Check sheet for the modelled part. Datum: model origin and axes. Units: mm. A direction names the side the tool comes from. Coordinates: 2 decimals unless noted, no trailing zeros. Loops run counter-clockwise (first coordinate to the right, second up) from the corner with the lowest first, then second, coordinate; pieces in that order, holes last. Notation, with made-up numbers: M 68.5,72 L 75.5,72 A9 ccw 75.5,79 Z; hole C 80,80 d10. An arc over 180 degrees is marked long. Return JSON: item names as keys, results as strings.
from build123d import *

# Parameters (mm, degrees)
SKETCH1_W           = 285
SKETCH1_H           = 36
SKETCH1_R           = 1.5
SKETCH1_W_2         = 42
SKETCH1_H_2         = 20
BOSS_EXTRUDE2_DEPTH = 5
FILLET1_R           = 6
FILLET2_R           = 1


with BuildPart() as part:
    # Sketch1 → Boss-Extrude2 (new body)
    with BuildSketch(Plane(origin=(0, 0, 0), x_dir=(1, 0, 0), z_dir=(0, 1, 0))):
        Rectangle(SKETCH1_W, SKETCH1_H)
        with Locations(Location((-22.5, -12, 0), (0, 0, 270))):
            Circle(SKETCH1_R, mode=Mode.SUBTRACT)
        with Locations(Location((-22.5, 12, 0), (0, 0, 90))):
            Circle(SKETCH1_R, mode=Mode.SUBTRACT)
        with Locations(Location((-136.5, -12, 0), (0, 0, 270))):
            Circle(SKETCH1_R, mode=Mode.SUBTRACT)
        with Locations(Location((-136.5, 12, 0), (0, 0, 90))):
            Circle(SKETCH1_R, mode=Mode.SUBTRACT)
        with Locations(Location((22.5, -12, 0), (0, 0, 90))):
            Circle(SKETCH1_R, mode=Mode.SUBTRACT)
        with Locations(Location((22.5, 12, 0), (0, 0, 270))):
            Circle(SKETCH1_R, mode=Mode.SUBTRACT)
        with Locations(Location((136.5, -12, 0), (0, 0, 90))):
            Circle(SKETCH1_R, mode=Mode.SUBTRACT)
        with Locations(Location((136.5, 12, 0), (0, 0, 270))):
            Circle(SKETCH1_R, mode=Mode.SUBTRACT)
        with Locations(Location((-60, 12, 0), (0, 0, 270))):
            Circle(SKETCH1_R, mode=Mode.SUBTRACT)
        with Locations(Location((-60, -12, 0), (0, 0, 90))):
            Circle(SKETCH1_R, mode=Mode.SUBTRACT)
        with Locations(Location((60, -12, 0), (0, 0, 270))):
            Circle(SKETCH1_R, mode=Mode.SUBTRACT)
        with Locations(Location((60, 12, 0), (0, 0, 90))):
            Circle(SKETCH1_R, mode=Mode.SUBTRACT)
        with Locations((-109, 0)):
            Rectangle(SKETCH1_W_2, SKETCH1_H_2, mode=Mode.SUBTRACT)
        with Locations((109, 0)):
            Rectangle(SKETCH1_W_2, SKETCH1_H_2, mode=Mode.SUBTRACT)
    extrude(amount=BOSS_EXTRUDE2_DEPTH)

    # Fillet1
    fillet1_edges = [part.edges().sort_by_distance(p)[0] for p in [
        (142.5, 2.5, 18),
        (-142.5, 2.5, 18),
        (-142.5, 2.5, -18),
        (142.5, 2.5, -18),
    ]]
    fillet(fillet1_edges, radius=FILLET1_R)

    # Fillet2
    fillet2_edges = [part.edges().sort_by_distance(p)[0] for p in [
        (-88, 2.5, 10),
        (-88, 2.5, -10),
        (-130, 2.5, -10),
        (-130, 2.5, 10),
        (88, 2.5, -10),
        (88, 2.5, 10),
        (130, 2.5, 10),
        (130, 2.5, -10),
    ]]
    fillet(fillet2_edges, radius=FILLET2_R)


solid = part.part
1) Set-up check for faces 5 (the face through (142.5, 2, 0)), 6 (the face through (-88, 2, 0)): record each of +Z, -Z, +X, -X, +Y, -Y from which the full face is reachable in a straight line by a thin tool's end or side.
Answers:
{"face 5": "+Z, -Z, +X, +Y, -Y", "face 6": "+Y, -Y"}
2) Draft check along Z on faces 1 (the face through (-2, 0, 0)), 2 (the face through (140.696, 2.535, 16.289)), 3 (the face through (-109, 2, -10)), 4 (the face through (109, 2, 10)). Enter one of: +Z half, -Z half, draft (parallel to the pull), parting line (faces both ways), or undercut.
Answers:
{"face 1": "draft", "face 2": "+Z half", "face 3": "undercut", "face 4": "undercut"}
3) Section check A-A on x = -96. Record the cut outline in (y, z).
Answers:
{"outline": "M 0,-18 L 5,-18 L 5,-10 L 0,-10 Z; M 0,10 L 5,10 L 5,18 L 0,18 Z"}
4) Scan lines: line 1 along X through (y, z) = (0.45, 7); line 2 along Z through (x, y) = (136.5, 3.55); line 3 along Z through (x, y) = (-116, 0.85). Record each from-to range of solid material in increasing order. Write a range as [from, to].
Answers:
{"line 1": "[-142.5, -130], [-88, 88], [130, 142.5]", "line 2": "[-18, -13.5], [-10.5, 10.5], [13.5, 18]", "line 3": "[-18, -10], [10, 18]"}
5) Go/stop test with flat-tipped pins: pin 1 Ø1.8 at (x, z) = (-136.5, -12) entering from -Y; pin 2 Ø5 at (x, z) = (136.5, 12) entering from -Y. Record where each tip stops, or that it passes through.
Answers:
{"pin 1": "through", "pin 2": "y = 0"}
6) Section check B-B on y = 3.3. Count the separate pieces of the cut face and the enclosed holes in it, then the cut area to 3 significant figures.
Answers:
{"separate pieces": "1", "enclosed holes": "14", "area": "8,470 mm²"}
